```python
from build123d import *

# Parameters (mm, degrees)
F1_DEPTH = 3
F3_DEPTH = 70
F4_R     = 1.9
F4_R_2   = 4.05
F5_DEPTH = 4


# Not quite as in the source:
# - a feature names something its author has since deleted; it is built from what else it names


with BuildPart() as f1:
    # F0 (on Top) → F1 (new body)
    with BuildSketch(Plane.XY):
        with BuildLine():
            Line((14, 13), (-14, 13))
            ThreePointArc((-14, 13), (-19.3340623478, 0), (-14, -13))
            Line((-14, -13), (14, -13))
            ThreePointArc((14, -13), (19.3340623478, 0), (14, 13))
        make_face()
    extrude(amount=F1_DEPTH)

    # F2 (on face) → F3 (join)
    with BuildSketch(Plane.XY.offset(3)):
        with BuildLine():
            ThreePointArc((14, -13), (19.3340623478, 0), (14, 13))
            Line((14, 13), (-14, 13))
            ThreePointArc((-14, 13), (-19.3340623478, 0), (-14, -13))
            Line((-14, -13), (14, -13))
        make_face()
        with BuildLine():
            Line((13.4202267877, -11.5), (-13.4202267877, -11.5))
            ThreePointArc((-13.4202267877, -11.5), (-17.8340623478, 0), (-13.4202267877, 11.5))
            Line((-13.4202267877, 11.5), (13.4202267877, 11.5))
            ThreePointArc((13.4202267877, 11.5), (17.8340623478, 0), (13.4202267877, -11.5))
        make_face(mode=Mode.SUBTRACT)
    extrude(amount=F3_DEPTH)

    # F4 (on face) → F5 (cut)
    with BuildSketch(Plane.XZ.offset(13)):
        with Locations((-8, 35)):
            Circle(F4_R)
        with Locations((0, 35)):
            Circle(F4_R_2)
        with Locations((8, 35)):
            Circle(F4_R)
        with Locations((0, 43)):
            Circle(F4_R)
        with Locations((0, 27)):
            Circle(F4_R)
    extrude(amount=-F5_DEPTH, mode=Mode.SUBTRACT)


solid = f1.part
```
Verification items for the finished model (mm, model axes). A direction names the side the tool comes from. Give positions to 0.01 mm unless a question says otherwise; leave off trailing zeros. Loops run counter-clockwise (first coordinate to the right, second up) from the corner with the lowest first, then second, coordinate; pieces in that order, holes last.
1. Mould release check, pull along X, two halves, no side actions. Record for faces 4 (the cylindrical face through (-19.333, 0.202, 35.989)), 5 (the cylindrical face through (-8.412, -12.26, 33.145)), 6 (the flat face through (6, -13, 36)), 7 (the cylindrical face through (19.333, -0.202, 35.989)): released by +X, released by -X, zero draft, split by the parting line, or undercut.
2. Section check C-C, the plane z = 16. Enter the section's corners in (x, y), then the cut area to 3 significant figures.
3. Go/stop test with flat-tipped pins: pin 1 Ø12 at (y, z) = (10, 59) entering from +X; pin 2 Ø2 at (y, z) = (-4, 17.5) entering from -X; pin 3 Ø4 at (x, y) = (1, 7) entering from +Z. Record where each tip stops, or that it passes through.
4. Section check D-D, the plane z = 35. Enter the section's corners in (x, y), then the cut area to 3 significant figures.
5. Section check A-A, the plane x = 0. Enter the section's corners in (y, z).
6. Set-up check for faces 1 (the flat face through (0, 11.5, 38)), 2 (the cylindrical face through (-0.247, -12.26, 28.884)), 3 (the flat face through (0, 12, 73)): record each of +Z, -Z, +X, -X, +Y, -Y from which the full face is reachable in a straight line by a thin tool's end or side.
7. Section check B-B, the plane x = 8. Enter the section's corners in (y, z).
8. Thickness scan on line 1 (Z direction, x = 0, y = -12.6); line 2 (Y direction, x = 5, z = 12); line 3 (Z direction, x = -8, y = -12.2). Record the ranges inside material, lowest first.
Geometry says:
1. face 4: released by -X
1. face 5: undercut
1. face 6: zero draft
1. face 7: released by +X
2. outline: (-14, -13) - (14, -13) arc R18.51 ccw to (14, 13) - (-14, 13) arc R18.51 ccw to start; hole (-13.42, -11.5) - (13.42, -11.5) arc R17.19 ccw to (13.42, 11.5) - (-13.42, 11.5) arc R17.19 ccw to start
2. area: 162 mm2
3. pin 1: stops at x = 18.9
3. pin 2: stops at x = -19.09
3. pin 3: stops at z = 3
4. outline: (-14, -13) - (-9.9, -13) - (-9.9, -11.5) - (-13.42, -11.5) arc R17.19 cw to (-13.42, 11.5) - (13.42, 11.5) arc R17.19 cw to (13.42, -11.5) - (9.9, -11.5) - (9.9, -13) - (14, -13) arc R18.51 ccw to (14, 13) - (-14, 13) arc R18.51 ccw to start; (-6.1, -13) - (-4.05, -13) - (-4.05, -11.5) - (-6.1, -11.5) - close; (4.05, -13) - (6.1, -13) - (6.1, -11.5) - (4.05, -11.5) - close
4. area: 139 mm2
5. outline: (-13, 0) - (13, 0) - (13, 73) - (11.5, 73) - (11.5, 3) - (-11.5, 3) - (-11.5, 25.1) - (-13, 25.1) - close; (-13, 28.9) - (-11.5, 28.9) - (-11.5, 30.95) - (-13, 30.95) - close; (-13, 39.05) - (-11.5, 39.05) - (-11.5, 41.1) - (-13, 41.1) - close; (-13, 44.9) - (-11.5, 44.9) - (-11.5, 73) - (-13, 73) - close
6. face 1: +Z
6. face 2: -Y
6. face 3: +Z, +X, -X, +Y, -Y
7. outline: (-13, 0) - (13, 0) - (13, 73) - (11.5, 73) - (11.5, 3) - (-11.5, 3) - (-11.5, 33.1) - (-13, 33.1) - close; (-13, 36.9) - (-11.5, 36.9) - (-11.5, 73) - (-13, 73) - close
8. line 1: z = 0 to 25.1, 28.9 to 30.95, 39.05 to 41.1, 44.9 to 73
8. line 2: y = -13 to -11.5, 11.5 to 13
8. line 3: z = 0 to 33.1, 36.9 to 73
